Autodesk Inventor part; units mm, degrees
ref_plane "YZ Plane" through (0, 0, 0) normal (1, 0, 0) x (0, 1, 0)
ref_plane "XZ Plane" through (0, 0, 0) normal (0, 1, 0) x (-1, 0, 0)
ref_plane "XY Plane" through (0, 0, 0) normal (0, 0, 1) x (1, 0, 0)
sketch "Esquisse1" plane through (0, 0, 0) normal (0, 0, 1) x (1, 0, 0)
  line L0 (0, 0) -> (90, 0)
  line L1 (90, 0) -> (90, 67)
  line L2 (90, 67) -> (0, 67)
  line L3 (0, 67) -> (0, 0)
  dimension "d0" = 90
  dimension "d1" = 67
extrude "Extrusion1" add sketch "Esquisse1" along normal blind 10
sketch "Esquisse2" plane through (0, 0, 10) normal (0, 0, 1) x (1, 0, 0)
  circle A0 centre (15, 20) radius 13
  line L0 (0, 0) -> (90, 0)
  line L1 (0, 67) -> (0, 0)
  circle A1 centre (75, 15) radius 13
  line L2 (90, 0) -> (90, 67)
  circle A2 centre (15, 29.9) radius 1.1
  circle A3 centre (5.1, 20) radius 1.1
  circle A4 centre (15, 10.1) radius 1.1
  circle A5 centre (24.9, 20) radius 1.1
  circle A6 centre (15, 20) radius 2.75
  dimension "d4" = 26
  dimension "d5" = 20
  dimension "d6" = 15
  dimension "d7" = 26
  dimension "d8" = 15
  dimension "d9" = 15
  dimension "d10" = 2.2
  dimension "d11" = 2
  dimension "d12" = 15
  dimension "d15" = 360
  dimension "d17" = 5.5
extrude "Extrusion2" cut sketch "Esquisse2" against normal blind 10 contours A2 | A3 | A4 | A5 | A6
sketch "Esquisse3" plane through (0, 0, 10) normal (0, 0, 1) x (1, 0, 0)
  circle A0 centre (45, 22) radius 11
  line L0 (0, 0) -> (90, 0)
  line L1 (90, 0) -> (90, 67)
  dimension "d20" = 22
  dimension "d21" = 45
  dimension "d22" = 22
extrude "Extrusion3" cut sketch "Esquisse3" against normal blind 10
sketch "Esquisse4" plane through (0, 0, 10) normal (0, 0, 1) x (1, 0, 0)
  circle A0 centre (15, 20) radius 2.75
  circle A1 centre (15, 20) radius 13
  point P0 (0, 0)
  dimension "d25" = 26
extrude "Extrusion4" cut sketch "Esquisse4" against normal blind 5
properties part number "Flancs"
The model under review builds one solid part; all positions refer to its coordinate system, in mm. A direction names the side the tool comes from. Give positions to 0.01 mm unless a question says otherwise; leave off trailing zeros. Loops run counter-clockwise (first coordinate to the right, second up) from the corner with the lowest first, then second, coordinate; pieces in that order, holes last. Notation, with made-up numbers: (75, -23) -> (79, -23) arc R34 cw to (79, 15) -> close; hole circle Ø9 at (73, 6). An arc over 180 degrees is marked (long way). Answer as a JSON object with one key per item and string values. Group by question number.
Q1. Insertion check: pin 1 (1.8 mm diameter, centred on x = 15, y = 29.9, fed in from +Z); pin 2 (2.5 mm diameter, centred on x = 5.1, y = 20, fed in from +Z). Each pin has a flat end and moves straight along its axis. Give the tip position at first contact, or say it passes through.
Q2. Take a section at B-B (z = 3). Write out the cut boundary in (x, y).
Q3. Take a section at D-D (z = 8.75). Write out the cut boundary in (x, y), plus the area to 3 significant figures.
Q4. Draft analysis for pull direction X (two halves, no side actions). For faces 1 (the flat face through (90, 33, 5)), 2 (the cylindrical face through (25.408, 19.024, 2.535)), 3 (the flat face through (44, 0, 5)), 4 (the flat face through (0, 34, 5)), state which applies: pulls with the +X half, pulls with the -X half, needs draft (parallel to the pull), parting line crosses it, or undercut.
Q5. Take a section at C-C (x = 24.9). Write out the cut boundary in (y, z), plus the area to 3 significant figures.
Q6. Take a section at A-A (x = 15). Write out the cut boundary in (y, z).
Q7. Wall thickness on line 1 along Y through (x, z) = (15, 1.4); line 2 along Y through (x, z) = (5.1, 2.95); line 3 along X through (y, z) = (31, 9): over which ranges is each line inside the solid? List them lowest first.
Q8. Tool access review of faces 5 (the flat face through (15, 23, 5)), 6 (the flat face through (44, 34, 0)): name each direction out of +Z, -Z, +X, -X, +Y, -Y from which nothing blocks a thin tool from reaching the whole face with its end or side.
Answer below:
{
 "1": {"pin 1": "passes through", "pin 2": "stops at z = 5"},
 "2": {"outline": "(0, 0) -> (90, 0) -> (90, 67) -> (0, 67) -> close; hole circle Ø2.2 at (5.1, 20); hole circle Ø5.5 at (15, 20); hole circle Ø2.2 at (15, 10.1); hole circle Ø2.2 at (15, 29.9); hole circle Ø2.2 at (24.9, 20); hole circle Ø22 at (45, 22)"},
 "3": {"outline": "(0, 0) -> (90, 0) -> (90, 67) -> (0, 67) -> close; hole circle Ø26 at (15, 20); hole circle Ø22 at (45, 22)", "area": "5,120 mm2"},
 "4": {"face 1": "pulls with the +X half", "face 2": "undercut", "face 3": "needs draft", "face 4": "pulls with the -X half"},
 "5": {"outline": "(0, 0) -> (18.9, 0) -> (18.9, 5) -> (11.57, 5) -> (11.57, 10) -> (0, 10) -> close; (21.1, 0) -> (67, 0) -> (67, 10) -> (28.43, 10) -> (28.43, 5) -> (21.1, 5) -> close", "area": "575 mm2"},
 "6": {"outline": "(0, 0) -> (9, 0) -> (9, 5) -> (7, 5) -> (7, 10) -> (0, 10) -> close; (11.2, 0) -> (17.25, 0) -> (17.25, 5) -> (11.2, 5) -> close; (22.75, 0) -> (28.8, 0) -> (28.8, 5) -> (22.75, 5) -> close; (31, 0) -> (67, 0) -> (67, 10) -> (33, 10) -> (33, 5) -> (31, 5) -> close"},
 "7": {"line 1": "y = 0 to 9, 11.2 to 17.25, 22.75 to 28.8, 31 to 67", "line 2": "y = 0 to 18.9, 21.1 to 67", "line 3": "x = 0 to 8.07, 21.93 to 38.68, 51.32 to 90"},
 "8": {"face 5": "+Z", "face 6": "-Z, +X, -X, +Y, -Y"}
}
